Work out the finished part from the listing and answer in its coordinate system (mm). Face numbers are marked on the shaded views. Round coordinates to 2 decimals unless told otherwise and drop trailing zeros. Loops run counter-clockwise (first coordinate to the right, second up) from the corner with the lowest first, then second, coordinate; pieces in that order, holes last. Notation, with made-up numbers: (39.5, 20) -> (77.5, 20) arc R18 cw to (77.5, 50) -> close; hole circle Ø4 at (-1.5, 6). An arc over 180 degrees is marked (long way). Use one line per item in the form item = value.
Autodesk Inventor part; units mm, degrees
ref_plane "YZ Plane" through (0, 0, 0) normal (1, 0, 0) x (0, 1, 0)
ref_plane "XZ Plane" through (0, 0, 0) normal (0, 1, 0) x (-1, 0, 0)
ref_plane "XY Plane" through (0, 0, 0) normal (0, 0, 1) x (1, 0, 0)
sketch "스케치1" plane through (0, 0, 0) normal (0, 1, 0) x (-1, 0, 0)
  arc A0 (0, 0) -> (17.6777, -17.6777) centre (17.9972, 0.3195) ccw
  line L0 (0, 0) -> (17.6777, -17.6777) construction
  line L1 (0, 0) -> (25, 0) construction
  arc A1 (-0.898, 2.3123) -> (19.9899, -18.5757) centre (17.9972, 0.3195) ccw
  line L2 (-0.898, 2.3123) -> (19.9899, -18.5757)
  line L3 (0, 0) -> (0, 1.4142)
  line L4 (17.6777, -17.6777) -> (19.0919, -17.6777)
  dimension "d0" = 25
  dimension "d1" = 45
  dimension "d2" = 18
  dimension "d3" = 1
extrude "돌출1" add sketch "스케치1" along normal blind 90 contours A0 L4 L2 A1 L3
sketch "스케치2" plane through (0, 0, 0) normal (0, -1, 0) x (1, 0, 0)
  circle A0 centre (-19.0919, -14.6777) radius 1.5
  arc A1 (-17.6777, -17.6777) -> (0, 0) centre (-17.9972, 0.3195) ccw
  circle A2 centre (-19.0919, -14.6777) radius 2.5
  line L0 (-19.0919, -12.1777) -> (-5.0426, -12.1777)
  line L1 (-21.5919, -14.6777) -> (-21.5919, -18.2148)
  line L2 (-21.5919, -14.6777) -> (-18.0548, -14.6777) construction
  line L3 (-19.9899, -18.5757) -> (-19.0919, -17.6777)
  line L4 (-19.9899, -18.5757) -> (-21.5919, -18.5757)
  line L5 (-21.5919, -18.5757) -> (-21.5919, -18.2148)
  line L6 (0, 0) -> (0, 1.4142)
  line L7 (0, 1.4142) -> (0.898, 2.3123)
  arc A3 (-19.9899, -18.5757) -> (0.898, 2.3123) centre (-17.9972, 0.3195) ccw
  line L8 (-19.9899, -18.5757) -> (-19.0919, -17.6777)
  line L9 (-19.0919, -17.6777) -> (-17.6777, -17.6777)
  arc A4 (-17.6777, -17.6777) -> (0, 0) centre (-17.9972, 0.3195) ccw
  point P0 (-17.6777, -17.6777)
  dimension "d6" = 3
  dimension "d7" = 3
  dimension "d8" = 1
  dimension "d9" = 90
extrude "돌출2" add sketch "스케치2" against normal blind 3 contours L9 L3 L4 L5 L1 A2 L0 A1 | A2
fillet "모깎기1" radius 2 1 edges at (-21.5919, 1.5, -18.5757)
sketch "스케치3" plane through (0, 90, 0) normal (0, 1, 0) x (1, 0, 0)
  arc A0 (-19.9899, 18.5757) -> (-21.5919, 16.6157) centre (-19.5919, 16.6157) ccw
  line L0 (-21.5919, 16.6157) -> (-21.5919, 14.6777)
  arc A1 (-21.5919, 14.6777) -> (-19.0919, 12.1777) centre (-19.0919, 14.6777) ccw
  line L1 (-19.0919, 12.1777) -> (-5.0426, 12.1777)
  arc A2 (-5.0426, 12.1777) -> (-17.6777, 17.6777) centre (-17.9972, -0.3195) ccw
  line L2 (-19.0919, 17.6777) -> (-17.6777, 17.6777)
  line L3 (-19.9899, 18.5757) -> (-19.0919, 17.6777)
  circle A3 centre (-19.0919, 14.6777) radius 1.5
  point P0 (0, 0)
extrude "돌출3" add sketch "스케치3" against normal blind 3
properties part number "wind blade"
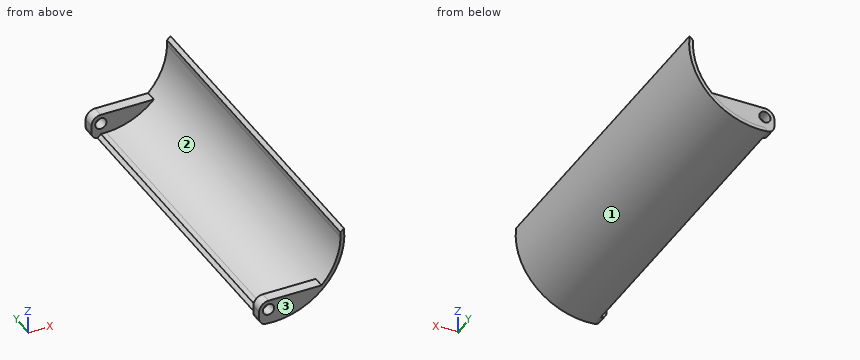
(1) Find section C-C, the plane z = -6.75. Write down the section's boundary in (x, y), then the cut area to 3 significant figures.
Completed:
outline = (-1.44, 0) -> (-0.36, 0) -> (-0.36, 90) -> (-1.44, 90) -> close
area = 97.4 mm2
(2) Consider L1, parallel to Y at x = -19.5, z = -12.25; L2, parallel to X at y = 51, z = -0.25; L3, parallel to X at y = 50, z = -10.5. Determine where each line is inside the solid, lowest interval first.
Completed:
L1 = 0 to 3, 87 to 90
L2 = -0.01 to 0.99
L3 = -3.61 to -2.38
(3) Find section A-A, the plane x = -11.5. Write down the section's boundary in (y, z), then the cut area to 3 significant figures.
Completed:
outline = (0, -17.54) -> (90, -17.54) -> (90, -12.18) -> (87, -12.18) -> (87, -16.47) -> (3, -16.47) -> (3, -12.18) -> (0, -12.18) -> close
area = 122 mm2
(4) Find section B-B, the plane y = 52.5. Write down the section's boundary in (x, z), then the cut area to 3 significant figures.
Completed:
outline = (-19.99, -18.58) arc R19 ccw to (0.9, 2.31) -> (0, 1.41) -> (0, 0) arc R18 cw to (-17.68, -17.68) -> (-19.09, -17.68) -> close
area = 32.1 mm2
(5) For a pull along Y with two mould halves and no side action, classify the marked faces 1, 2 and 3 as +Y half, -Y half, draft (parallel to the pull), parting line (faces both ways), or undercut.
Completed:
face_1 = draft
face_2 = undercut
face_3 = -Y half
(6) Given P1, Ø4, axis at x = -4.5, z = -5.5, coming from the -Y side; P2, Ø0.9, axis at x = -10.5, y = 1, coming from the +Z side; P3, Ø1.6, axis at x = -18, y = 34.5, coming from the +Z side; P4, Ø0.7, axis at y = 35, z = 1, coming from the -X side, each flat-ended and moving along its own axis, determine where each tip first touches the part or whether it passes through.
Completed:
P1 = through
P2 = -12.18
P3 = -17.66
P4 = 0
